from build123d import *

# Parameters (mm, degrees)
F0_R         = 11
F0_R_2       = 15
F1_DEPTH     = 20
F2_DEPTH     = 10
F3_T1_DEPTH  = 10
F3_T3_DEPTH  = 10
F3_T5_DEPTH  = 20
F3_T10_ANGLE = 38.1317076079
F3_T15_ANGLE = 38.1317076079
F3_T20_ANGLE = 38.1317076079
F3_T25_ANGLE = 38.1317076079
F3_T31_DEPTH = 18.0325080763
F3_T35_ANGLE = 38.1317076079
F3_T42_DEPTH = 18.0325080763
F3_T46_ANGLE = 38.1317076079
F3_T53_DEPTH = 18.0325080763
F3_T57_ANGLE = 38.1317076079
F3_T64_DEPTH = 18.0325080763
F3_T68_ANGLE = 38.1317076079


# Not quite as in the source:
# - a fillet or chamfer that OpenCascade refuses, or shapes differently, is made with other operations: its cross-section is extruded or revolved along the edge and cut away or added


with BuildPart() as f1:
    # F0 (on Front) → F1 (new body, symmetric)
    with BuildSketch(Plane.XZ):
        with BuildLine():
            ThreePointArc((45.8257569496, -20), (48.9453156465, -10.2154821845), (50, 0))
            ThreePointArc((50, 0), (48.9453156465, 10.2154821845), (45.8257569496, 20))
            ThreePointArc((45.8257569496, 20), (-50, 0), (45.8257569496, -20))
        make_face()
        with Locations((-28.145825623, -16.25)):
            Circle(F0_R, mode=Mode.SUBTRACT)
        with Locations((0, -32.5)):
            Circle(F0_R, mode=Mode.SUBTRACT)
        with Locations((28.145825623, -16.25)):
            Circle(F0_R, mode=Mode.SUBTRACT)
        with Locations((-28.145825623, 16.25)):
            Circle(F0_R, mode=Mode.SUBTRACT)
        Circle(F0_R_2, mode=Mode.SUBTRACT)
        with Locations((28.145825623, 16.25)):
            Circle(F0_R, mode=Mode.SUBTRACT)
        with Locations((0, 32.5)):
            Circle(F0_R, mode=Mode.SUBTRACT)
    extrude(amount=F1_DEPTH, both=True)

    # F0 (on Front) → F2 (join, symmetric)
    with BuildSketch(Plane.XZ):
        with BuildLine():
            ThreePointArc((45.8257569496, -20), (48.9453156465, -10.2154821845), (50, 0))
            ThreePointArc((50, 0), (48.9453156465, 10.2154821845), (45.8257569496, 20))
            ThreePointArc((45.8257569496, 20), (-50, 0), (45.8257569496, -20))
        make_face()
        with Locations((-28.145825623, -16.25)):
            Circle(F0_R, mode=Mode.SUBTRACT)
        with Locations((0, -32.5)):
            Circle(F0_R, mode=Mode.SUBTRACT)
        with Locations((28.145825623, -16.25)):
            Circle(F0_R, mode=Mode.SUBTRACT)
        with Locations((-28.145825623, 16.25)):
            Circle(F0_R, mode=Mode.SUBTRACT)
        Circle(F0_R_2, mode=Mode.SUBTRACT)
        with Locations((28.145825623, 16.25)):
            Circle(F0_R, mode=Mode.SUBTRACT)
        with Locations((0, 32.5)):
            Circle(F0_R, mode=Mode.SUBTRACT)
        with BuildLine():
            ThreePointArc((45.8257569496, 20), (48.9453156465, 10.2154821845), (50, 0))
            ThreePointArc((50, 0), (48.9453156465, -10.2154821845), (45.8257569496, -20))
            Line((45.8257569496, -20), (91.6475165291, -20))
            ThreePointArc((91.6475165291, -20), (83.8557409084, -45.8703249329), (70.2430836554, -69.2087276625))
            ThreePointArc((70.2430836554, -69.2087276625), (74.1794933933, -97.2177383265), (102.1885040573, -93.2813285886))
            ThreePointArc((102.1885040573, -93.2813285886), (133.4, 0), (102.1885040573, 93.2813285886))
            ThreePointArc((102.1885040573, 93.2813285886), (74.1794933933, 97.2177383265), (70.2430836554, 69.2087276625))
            ThreePointArc((70.2430836554, 69.2087276625), (83.8557409084, 45.8703249329), (91.6475165291, 20))
            Line((91.6475165291, 20), (45.8257569496, 20))
        make_face()
        with BuildLine():
            ThreePointArc((94.2021489569, -87.263178357), (80.1976436249, -89.231383226), (78.2294387559, -75.226877894))
            ThreePointArc((78.2294387559, -75.226877894), (103.4, 0), (78.2294387559, 75.226877894))
            ThreePointArc((78.2294387559, 75.226877894), (80.1976436249, 89.231383226), (94.2021489569, 87.263178357))
            ThreePointArc((94.2021489569, 87.263178357), (123.4, 0), (94.2021489569, -87.263178357))
        make_face(mode=Mode.SUBTRACT)
    extrude(amount=F2_DEPTH, both=True)

    # F3: fillet of radius 5.08 on 10 edges, made by hand

    # F3_s2 → F3_t1 (join)
    with BuildSketch(Plane.XZ.offset(-10)):
        with BuildLine():
            ThreePointArc((44.5159406137, 22.7668845316), (46.3877440145, 20.7465818007), (49.0387601801, 20))
            Line((49.0387601801, 20), (45.8257569496, 20))
            ThreePointArc((45.8257569496, 20), (45.1920290777, 21.3934688128), (44.5159406137, 22.7668845316))
        make_face()
        with BuildLine():
            ThreePointArc((44.5159406137, -22.7668845316), (46.3877440145, -20.7465818007), (49.0387601801, -20))
            Line((49.0387601801, -20), (45.8257569496, -20))
            ThreePointArc((45.8257569496, -20), (45.1920290777, -21.3934688128), (44.5159406137, -22.7668845316))
        make_face()
    extrude(amount=F3_T1_DEPTH)

    # F3_s4 → F3_t3 (join)
    with BuildSketch(Plane.XZ):
        with BuildLine():
            ThreePointArc((44.5159406137, 22.7668845316), (46.3877440145, 20.7465818007), (49.0387601801, 20))
            Line((49.0387601801, 20), (45.8257569496, 20))
            ThreePointArc((45.8257569496, 20), (45.1920290777, 21.3934688128), (44.5159406137, 22.7668845316))
        make_face()
        with BuildLine():
            ThreePointArc((44.5159406137, -22.7668845316), (46.3877440145, -20.7465818007), (49.0387601801, -20))
            Line((49.0387601801, -20), (45.8257569496, -20))
            ThreePointArc((45.8257569496, -20), (45.1920290777, -21.3934688128), (44.5159406137, -22.7668845316))
        make_face()
    extrude(amount=F3_T3_DEPTH)

    # F3_s6 → F3_t5 (join)
    with BuildSketch(Plane.XZ.offset(-10)):
        with BuildLine():
            ThreePointArc((85.4205587726, -20), (89.4014218376, -21.924191188), (90.3665598512, -26.2390829694))
            ThreePointArc((90.3665598512, -26.2390829694), (91.0502400753, -23.1284113368), (91.6475165291, -20))
            Line((91.6475165291, -20), (85.4205587726, -20))
        make_face()
        with BuildLine():
            ThreePointArc((85.4205587726, 20), (89.4014218376, 21.924191188), (90.3665598512, 26.2390829694))
            ThreePointArc((90.3665598512, 26.2390829694), (91.0502400753, 23.1284113368), (91.6475165291, 20))
            Line((91.6475165291, 20), (85.4205587726, 20))
        make_face()
    extrude(amount=F3_T5_DEPTH)


with BuildPart() as f3_tool8:
    # F3_s9 → F3_t10 (revolve)
    with BuildSketch(Plane(origin=(0, 0, 0), x_dir=(0, 1, 0), z_dir=(-0.6174712722, 0, -0.7865934325))):
        with BuildLine():
            ThreePointArc((10, 55.08), (11.4878975516, 51.4878975516), (15.08, 50))
            Line((15.08, 50), (10, 50))
            Line((10, 50), (10, 55.08))
        make_face()
    revolve(axis=Axis((0, 10, 0), (0, -1, 0)), revolution_arc=F3_T10_ANGLE)

    split(bisect_by=Plane.XY.offset(-20), keep=Keep.TOP)


with BuildPart() as f1_1:
    add(f1.part)

    # F3_t7: union F3_tool8
    add(f3_tool8.part)


with BuildPart() as f3_tool13:
    # F3_s14 → F3_t15 (revolve)
    with BuildSketch(Plane.XY):
        with BuildLine():
            ThreePointArc((55.08, 10), (51.4878975516, 11.4878975516), (50, 15.08))
            Line((50, 15.08), (50, 10))
            Line((50, 10), (55.08, 10))
        make_face()
    revolve(axis=Axis((0, 10, 0), (0, -1, 0)), revolution_arc=F3_T15_ANGLE)

    split(bisect_by=Plane.XY.offset(20), keep=Keep.BOTTOM)


with BuildPart() as f1_2:
    add(f1_1.part)

    # F3_t12: union F3_tool13
    add(f3_tool13.part)


with BuildPart() as f3_tool18:
    # F3_s19 → F3_t20 (revolve)
    with BuildSketch(Plane.XY):
        with BuildLine():
            ThreePointArc((55.08, -10), (51.4878975516, -11.4878975516), (50, -15.08))
            Line((50, -15.08), (50, -10))
            Line((50, -10), (55.08, -10))
        make_face()
    revolve(axis=Axis((0, -10, 0), (0, 1, 0)), revolution_arc=F3_T20_ANGLE)

    split(bisect_by=Plane.XY.offset(-20), keep=Keep.TOP)


with BuildPart() as f1_3:
    add(f1_2.part)

    # F3_t17: union F3_tool18
    add(f3_tool18.part)


with BuildPart() as f3_tool23:
    # F3_s24 → F3_t25 (revolve)
    with BuildSketch(Plane(origin=(0, 0, 0), x_dir=(0, 1, 0), z_dir=(-0.6174712722, 0, 0.7865934325))):
        with BuildLine():
            ThreePointArc((-10, -55.08), (-11.4878975516, -51.4878975516), (-15.08, -50))
            Line((-15.08, -50), (-10, -50))
            Line((-10, -50), (-10, -55.08))
        make_face()
    revolve(axis=Axis((0, -10, 0), (0, 1, 0)), revolution_arc=F3_T25_ANGLE)

    split(bisect_by=Plane.XY.offset(20), keep=Keep.BOTTOM)


with BuildPart() as f1_4:
    add(f1_3.part)

    # F3_t22: union F3_tool23
    add(f3_tool23.part)


with BuildPart() as f3_tool29:
    # F3_s30 → F3_t31 (new body)
    with BuildSketch(Plane.XZ):
        with BuildLine():
            ThreePointArc((44.5159406137, 22.7668845316), (46.3877440145, 20.7465818007), (49.0387601801, 20))
            Line((49.0387601801, 20), (45.8257569496, 20))
            ThreePointArc((45.8257569496, 20), (45.1920290777, 21.3934688128), (44.5159406137, 22.7668845316))
        make_face()
    extrude(amount=-F3_T31_DEPTH)

    split(bisect_by=Plane.XZ.offset(-10), keep=Keep.BOTTOM)


with BuildPart() as f3_tool33:
    # F3_s34 → F3_t35 (revolve)
    with BuildSketch(Plane.XY):
        with BuildLine():
            ThreePointArc((55.08, 10), (51.4878975516, 11.4878975516), (50, 15.08))
            Line((50, 15.08), (50, 10))
            Line((50, 10), (55.08, 10))
        make_face()
    revolve(axis=Axis((0, 10, 0), (0, -1, 0)), revolution_arc=F3_T35_ANGLE)

    split(bisect_by=Plane.XY.offset(20), keep=Keep.TOP)


with BuildPart() as f3_tool29_1:
    add(f3_tool29.part)

    # F3_t37: intersect F3_tool33
    add(f3_tool33.part, mode=Mode.INTERSECT)


with BuildPart() as f1_5:
    add(f1_4.part)

    # F3_t27: union F3_tool29
    add(f3_tool29_1.part)


with BuildPart() as f3_tool40:
    # F3_s41 → F3_t42 (new body)
    with BuildSketch(Plane.XZ):
        with BuildLine():
            ThreePointArc((44.5159406137, 22.7668845316), (46.3877440145, 20.7465818007), (49.0387601801, 20))
            Line((49.0387601801, 20), (45.8257569496, 20))
            ThreePointArc((45.8257569496, 20), (45.1920290777, 21.3934688128), (44.5159406137, 22.7668845316))
        make_face()
    extrude(amount=F3_T42_DEPTH)

    split(bisect_by=Plane.XZ.offset(10), keep=Keep.TOP)


with BuildPart() as f3_tool44:
    # F3_s45 → F3_t46 (revolve)
    with BuildSketch(Plane(origin=(0, 0, 0), x_dir=(0, 1, 0), z_dir=(-0.6174712722, 0, 0.7865934325))):
        with BuildLine():
            ThreePointArc((-10, -55.08), (-11.4878975516, -51.4878975516), (-15.08, -50))
            Line((-15.08, -50), (-10, -50))
            Line((-10, -50), (-10, -55.08))
        make_face()
    revolve(axis=Axis((0, -10, 0), (0, 1, 0)), revolution_arc=F3_T46_ANGLE)

    split(bisect_by=Plane.XY.offset(20), keep=Keep.TOP)


with BuildPart() as f3_tool40_1:
    add(f3_tool40.part)

    # F3_t48: intersect F3_tool44
    add(f3_tool44.part, mode=Mode.INTERSECT)


with BuildPart() as f1_6:
    add(f1_5.part)

    # F3_t38: union F3_tool40
    add(f3_tool40_1.part)


with BuildPart() as f3_tool51:
    # F3_s52 → F3_t53 (new body)
    with BuildSketch(Plane.XZ):
        with BuildLine():
            ThreePointArc((44.5159406137, -22.7668845316), (46.3877440145, -20.7465818007), (49.0387601801, -20))
            Line((49.0387601801, -20), (45.8257569496, -20))
            ThreePointArc((45.8257569496, -20), (45.1920290777, -21.3934688128), (44.5159406137, -22.7668845316))
        make_face()
    extrude(amount=-F3_T53_DEPTH)

    split(bisect_by=Plane.XZ.offset(-10), keep=Keep.BOTTOM)


with BuildPart() as f3_tool55:
    # F3_s56 → F3_t57 (revolve)
    with BuildSketch(Plane(origin=(0, 0, 0), x_dir=(0, 1, 0), z_dir=(-0.6174712722, 0, -0.7865934325))):
        with BuildLine():
            ThreePointArc((10, 55.08), (11.4878975516, 51.4878975516), (15.08, 50))
            Line((15.08, 50), (10, 50))
            Line((10, 50), (10, 55.08))
        make_face()
    revolve(axis=Axis((0, 10, 0), (0, -1, 0)), revolution_arc=F3_T57_ANGLE)

    split(bisect_by=Plane.XY.offset(-20), keep=Keep.BOTTOM)


with BuildPart() as f3_tool51_1:
    add(f3_tool51.part)

    # F3_t59: intersect F3_tool55
    add(f3_tool55.part, mode=Mode.INTERSECT)


with BuildPart() as f1_7:
    add(f1_6.part)

    # F3_t49: union F3_tool51
    add(f3_tool51_1.part)


with BuildPart() as f3_tool62:
    # F3_s63 → F3_t64 (new body)
    with BuildSketch(Plane.XZ):
        with BuildLine():
            ThreePointArc((44.5159406137, -22.7668845316), (46.3877440145, -20.7465818007), (49.0387601801, -20))
            Line((49.0387601801, -20), (45.8257569496, -20))
            ThreePointArc((45.8257569496, -20), (45.1920290777, -21.3934688128), (44.5159406137, -22.7668845316))
        make_face()
    extrude(amount=F3_T64_DEPTH)

    split(bisect_by=Plane.XZ.offset(10), keep=Keep.TOP)


with BuildPart() as f3_tool66:
    # F3_s67 → F3_t68 (revolve)
    with BuildSketch(Plane.XY):
        with BuildLine():
            ThreePointArc((55.08, -10), (51.4878975516, -11.4878975516), (50, -15.08))
            Line((50, -15.08), (50, -10))
            Line((50, -10), (55.08, -10))
        make_face()
    revolve(axis=Axis((0, -10, 0), (0, 1, 0)), revolution_arc=F3_T68_ANGLE)

    split(bisect_by=Plane.XY.offset(-20), keep=Keep.BOTTOM)


with BuildPart() as f3_tool62_1:
    add(f3_tool62.part)

    # F3_t70: intersect F3_tool66
    add(f3_tool66.part, mode=Mode.INTERSECT)


with BuildPart() as f1_8:
    add(f1_7.part)

    # F3_t60: union F3_tool62
    add(f3_tool62_1.part)


solid = f1_8.part
Model file for the job. Use its own axes, mm. A direction names the side the tool comes from. Coordinates: 2 decimals unless noted, no trailing zeros. Write each loop counter-clockwise with the first axis right and the second up, starting at its lowest first coordinate (ties: lowest second). Pieces come first, ordered by that corner, then holes. Notation, with made-up numbers: (53.5, 79.5) -> (90.5, 79.5) arc R19 ccw to (90.5, 94.5) -> close; hole circle Ø8 at (10, 73). An arc over 180 degrees is marked (long way). One line per item, written item: value. Start each with the question number.
1) Pull direction X, two halves, no side cores. Call faces 3 (the face through (-12, -20, -10)), 4 (the face through (74.534, -0.14, 97.479)), 5 (the face through (67, 0, -20)): +X half, -X half, draft (parallel to the pull), parting line (faces both ways), or undercut.
2) Which spindle directions (+Z, -Z, +X, -X, +Y, -Y) get a long thin tool onto all of the face, cutting with end or side? Do faces 1 (the face through (82.686, -0.14, -48.47)), 2 (the face through (46.35, 0.21, 20.77)). Say none if no direction does.
3) Slice it at D-D on z = 0. Write the cut outline in (x, y), then the cut area to 3 significant figures.
4) Slice it at A-A on x = 0. Write the cut outline in (y, z), then the cut area to 3 significant figures.
5) Slice it at B-B on y = 6. Count the separate pieces of the cut face and the enclosed holes in it, then the cut area to 3 significant figures.
6) Probe probe 1 along Z at (x, y) = (0.5, 13.5); probe 2 along Z at (x, y) = (31.5, -17.5); probe 3 along X at (y, z) = (5.5, -9). List the from-to ranges inside material, lowest first.
7) Flat gauge pins, fed straight in: pin 1 Ø1 at (x, z) = (83, -19.5) entering from -Y; pin 2 Ø12 at (x, y) = (44, -6.5) entering from +Z; pin 3 Ø3 at (y, z) = (12.5, 30) entering from +X. Where does each tip first touch, or does it go through?
8) Slice it at C-C on z = -73. Write the cut outline in (x, y).
Answers follow:
1. face 3: draft
1. face 4: parting line
1. face 5: undercut
2. face 1: +Y, -Y
2. face 2: +Z, +Y, -Y
3. outline: (-50, -20) -> (-15, -20) -> (-15, 20) -> (-50, 20) -> close; (15, -20) -> (50, -20) -> (50, -15.08) arc R5.08 cw to (55.08, -10) -> (103.4, -10) -> (103.4, 10) -> (55.08, 10) arc R5.08 cw to (50, 15.08) -> (50, 20) -> (15, 20) -> close; (123.4, -10) -> (133.4, -10) -> (133.4, 10) -> (123.4, 10) -> close
3. area: 4,080 mm2
4. outline: (-20, -50) -> (20, -50) -> (20, -43.5) -> (-20, -43.5) -> close; (-20, -21.5) -> (20, -21.5) -> (20, -15) -> (-20, -15) -> close; (-20, 15) -> (20, 15) -> (20, 21.5) -> (-20, 21.5) -> close; (-20, 43.5) -> (20, 43.5) -> (20, 50) -> (-20, 50) -> close
4. area: 1,040 mm2
5. separate pieces: 1
5. enclosed holes: 8
5. area: 11,100 mm2
6. probe 1: -50 to -43.49, -21.51 to -14.99, 14.99 to 21.51, 43.49 to 50
6. probe 2: -38.83 to -26.73, -5.77 to 5.77, 26.73 to 38.83
6. probe 3: -49.18 to -36.42, -19.87 to -12, 12 to 19.87, 36.42 to 103.08, 123.12 to 133.14
7. pin 1: y = -10
7. pin 2: z = 32.5
7. pin 3: x = 41.08
8. outline: (67.99, -10) -> (79.87, -10) -> (79.87, 10) -> (67.99, 10) -> close; (103.68, -10) -> (115.13, -10) -> (115.13, 10) -> (103.68, 10) -> close
